Verification items for the finished model (mm, model axes). A direction names the side the tool comes from. Round coordinates to 2 decimals unless told otherwise and drop trailing zeros. Write each loop counter-clockwise with the first axis right and the second up, starting at its lowest first coordinate (ties: lowest second). Pieces come first, ordered by that corner, then holes. Notation, with made-up numbers: (57.25, -9.5) - (80.25, -9.5) arc R27 ccw to (80.25, 25.5) - close; hole circle Ø11 at (10.25, 44). An arc over 180 degrees is marked (long way). Answer as a JSON object with one key per item and string values. Group by question number.
1) Go/stop test with flat-tipped pins: pin 1 Ø12 at (y, z) = (-28, 195.5) entering from -X; pin 2 Ø1 at (x, y) = (47, -74.5) entering from +Z (3 decimals); pin 3 Ø1 at (y, z) = (126.5, -122.5) entering from -X. Record where each tip stops, or that it passes through.
2) Section check B-B (y = 61). Enter the section's corners in (x, z) (3 decimals), then the cut area to 3 significant figures.
3) Mould release check, pull along X, two halves, no side actions. Record for faces 1 (the flat face through (-12.05, 148.65, 563.63)), 2 (the flat face through (-95, 178, -701.675)), 3 (the flat face through (23.88, -140.58, -138.66)), 4 (the flat face through (0, -101, -130)): +X half, -X half, draft (parallel to the pull), parting line (faces both ways), or undercut.
4) Set-up check for faces 5 (the flat face through (-95, 179, -698.5)), 6 (the flat face through (3.175, -101, -128)), 7 (the flat face through (2, -27, 426.675)): record each of +Z, -Z, +X, -X, +Y, -Y from which the full face is reachable in a straight line by a thin tool's end or side.
5) Section check C-C (x = -267.5). Enter the section's corners in (y, z) (3 decimals).
6) Section check A-A (z = 529.5). Enter the section's corners in (x, y) (3 decimals), then the cut area to 3 significant figures.
7) Thickness scan on line 1 (Z direction, x = -237, y = 280.5) (3 decimals); line 2 (X direction, y = -16.5, z = -214.5) (3 decimals); line 3 (X direction, y = -107, z = -456). Record the ranges inside material, lowest first.
8) Section check D-D (z = 159.5). Enter the section's corners in (x, y) (3 decimals), then the cut area to 3 significant figures.
```python
from build123d import *

# Parameters (mm, degrees)
BOSS_EXTRUDE1_DEPTH = 701.675
SHELL1_T            = -3.175
SKETCH3_W           = 42
SKETCH3_H           = 290
CUT_EXTRUDE1_DEPTH  = 20
SKETCH7_W           = 275
SKETCH7_H           = 302.7
CUT_EXTRUDE5_DEPTH  = 100
CUT_EXTRUDE7_DEPTH  = 988.549739455
BOSS_EXTRUDE3_DEPTH = 6.35
BOSS_EXTRUDE4_DEPTH = 42
CHAMFER1_SIZE       = 7.134884114
CHAMFER1_SIZE_2     = 6.35


with BuildPart() as part:
    # Sketch2 → Boss-Extrude1 (new, symmetric)
    with BuildSketch(Plane.XY):
        Polygon((0, 0), (-105, 181.865334795), (-551.988806236, 244.144070894), (48.35, 350), (48.35, -200), (0, -200), align=None)
    extrude(amount=BOSS_EXTRUDE1_DEPTH, both=True)

    # Shell1
    shell1_openings = [part.faces().sort_by_distance(p)[0] for p in [
        (-251.819403118, 297.072035447, 0),
    ]]
    offset(amount=SHELL1_T, openings=shell1_openings, kind=Kind.INTERSECTION)

    # Sketch3 → Cut-Extrude1 (cut)
    with BuildSketch(Plane.XY.offset(701.675)):
        with Locations((24.175, -42.3)):
            Rectangle(SKETCH3_W, SKETCH3_H)
    extrude(amount=-CUT_EXTRUDE1_DEPTH, mode=Mode.SUBTRACT)

    # Sketch7 → Cut-Extrude5 (cut, symmetric)
    with BuildSketch(Plane.ZY):
        with Locations((564.175, -48.65)):
            Rectangle(SKETCH7_W, SKETCH7_H)
    extrude(amount=CUT_EXTRUDE5_DEPTH, both=True, mode=Mode.SUBTRACT)

    # Sketch9 → Cut-Extrude7 (cut, through all)
    with BuildSketch(Plane(origin=(48.35, 0, 0), x_dir=(0, 0, -1), z_dir=(1, 0, 0))):
        Polygon((-701.675, 102.7), (-426.675, 102.7), (-701.675, 181.7), align=None)
    extrude(amount=-CUT_EXTRUDE7_DEPTH, mode=Mode.SUBTRACT)

    # Sketch11 → Boss-Extrude3 (add)
    with BuildSketch(Plane(origin=(0, -18.35715529, 5.273510065), x_dir=(1, 0, 0), z_dir=(0, -0.9611272890955623, 0.27610565759472516))):
        Polygon((48.35, 724.567388561), (48.35, 438.44503711), (-59.293872646, 438.44503711), (-104.904543912, 724.567388561), align=None)
    extrude(amount=-BOSS_EXTRUDE3_DEPTH)

    # Sketch12 → Boss-Extrude4 (add)
    with BuildSketch(Plane(origin=(3.175, 0, 0), x_dir=(0, 0, -1), z_dir=(1, 0, 0))):
        Polygon((688.975, -79.565459926), (-396.466892858, -193.65), (-396.466892858, -196.825), (688.975, -82.740459926), align=None)
        Polygon((-396.466892858, -193.65), (-426.675, -196.825), (-396.466892858, -196.825), align=None)
    extrude(amount=BOSS_EXTRUDE4_DEPTH)

    # Chamfer1
    # the kernel refuses this chamfer: 7.134884114, 6.35 mm, written as the material it takes off along each edge
    with BuildSketch(Plane(origin=(3.175, -196.825, 426.675), x_dir=(0, -0.9997021141585574, 0.02440661686737172), z_dir=(1, 0, 0))) as chamfer1_piece_1:
        Polygon((CHAMFER1_SIZE * 0.999702114118, CHAMFER1_SIZE * 0.0244066168664), (-CHAMFER1_SIZE_2 * 0.128770240585, CHAMFER1_SIZE_2 * 0.991674455222), (0, 0), align=None)
    extrude(amount=42, mode=Mode.SUBTRACT)


solid = part.part
```
Returned:
{
 "1": {"pin 1": "x = 0", "pin 2": "z = 426.675", "pin 3": "x = -73.32"},
 "2": {"outline": "(-35.218, -701.675) - (48.35, -701.675) - (48.35, 426.675) - (45.175, 426.675) - (45.175, -698.5) - (-31.552, -698.5) - (-31.552, 426.675) - (-35.218, 426.675) - close", "area": "7,960 mm2"},
 "3": {"face 1": "undercut", "face 2": "draft", "face 3": "undercut", "face 4": "-X half"},
 "4": {"face 5": "+Y", "face 6": "none", "face 7": "+Z, +X, -X, -Y"},
 "5": {"outline": "(204.506, -701.675) - (294.307, -701.675) - (294.307, -698.5) - (207.712, -698.5) - (207.712, 698.5) - (294.307, 698.5) - (294.307, 701.675) - (204.506, 701.675) - close"},
 "6": {"outline": "(-551.989, 244.144) - (-105, 181.865) - (-76.348, 132.239) - (48.35, 132.239) - (48.35, 350) - (45.175, 349.44) - (45.175, 138.846) - (-76.496, 138.846) - (-103.026, 184.796) - (-541.833, 245.935) - close", "area": "3,090 mm2"},
 "7": {"line 1": "-701.675 to -698.5, 698.5 to 701.675", "line 2": "0 to 3.175, 45.175 to 48.35", "line 3": "0 to 48.35"},
 "8": {"outline": "(-551.989, 244.144) - (-105, 181.865) - (0, 0) - (0, -200) - (48.35, -200) - (48.35, 350) - (45.175, 349.44) - (45.175, -168.744) - (3.175, -168.744) - (3.175, 0.851) - (-103.026, 184.796) - (-541.833, 245.935) - close; hole (3.175, -196.825) - (45.175, -196.825) - (45.175, -171.919) - (3.175, -171.919) - close", "area": "4,740 mm2"}
}
